from build123d import *

# Parameters (mm, degrees)
F1_DEPTH = 38.1
F3_DEPTH = 60.292894
F5_R     = 5.25769
F5_W     = 14.030187
F5_H     = 4.162106
F6_DEPTH = 130.254248
F4_W     = 54.139016
F4_H     = 9.669455
F7_DEPTH = 60.292894


with BuildPart() as f1:
    # F0 (on Top) → F1 (new body)
    with BuildSketch(Plane.XY):
        Polygon((82.095571, 21.614075), (-48.157677, 21.614075), (-48.157677, -38.677819), (36.971442, -38.677819), (36.971442, -20.666091), (82.095571, -20.666091), align=None)
    extrude(amount=F1_DEPTH)

    # F2 (on face) → F3 (cut, through all)
    with BuildSketch(Plane.XZ.offset(38.677819)):
        Polygon((82.158446, 38.1), (28.353805, 38.1), (82.158446, 0), align=None)
    extrude(amount=-F3_DEPTH, mode=Mode.SUBTRACT)

    # F5 (on face) → F6 (cut, through all)
    with BuildSketch(Plane(origin=(-48.157677, 0, 0), x_dir=(0, -1, 0), z_dir=(-1, 0, 0))):
        with Locations((-14.877267, 31.217162)):
            Circle(F5_R)
        with Locations((-2.21119, 31.217162)):
            Circle(F5_R)
        with Locations((-2.990069, 19.638609)):
            Circle(F5_R)
        with Locations((-14.2001, 19.638609)):
            Circle(F5_R)
        with Locations((12.323814, 36.018947)):
            Rectangle(F5_W, F5_H)
    extrude(amount=-F6_DEPTH, mode=Mode.SUBTRACT)

    # F4 (on face) → F7 (cut, through all)
    with BuildSketch(Plane.XZ.offset(38.677819)):
        with Locations((-21.088169, 4.834727)):
            Rectangle(F4_W, F4_H)
    extrude(amount=-F7_DEPTH, mode=Mode.SUBTRACT)


solid = f1.part
Could you check a few things on this model? Use its own coordinates, in mm. A direction names the side the tool comes from. Coordinates: 2 decimals unless noted, no trailing zeros. Order: outer loops, then holes, each group sorted by start corner. A loop starts at its lowest first (then second) coordinate and runs counter-clockwise, first axis right, second up. Notation, with made-up numbers: (37, 49.25) - (86, 49.25) arc R12 ccw to (86, 56.25) - close; hole circle Ø5 at (10.5, 76.5). An arc over 180 degrees is marked (long way). Answer in a Markdown table with one row per item. Add a question column.
(1) On a 3-axis mill with a long thin cutter (end or side, diameter ignored), from which of +Z, -Z, +X, -X, +Y, -Y can I reach the whole of each face in a straight line? I mean faces 1 (the face through (54, -20.666, 12)), 2 (the face through (-21, -9, 9.669)), 3 (the face through (-8, -19.339, 36)). Say none if no direction works.
(2) Will these pins go through, and if not, where does the flat tip stop? pin 1 (1 mm diameter, centred on y = 4, z = 7, fed in from +X); pin 2 (11 mm diameter, centred on x = -19.5, y = -13.5, fed in from +Z); pin 3 (1 mm diameter, centred on x = 53, z = 20, fed in from -Y).
(3) If we section it at B-B, the plane x = 43.5: Please give me the cut outline in (y, z), then the cut area to 3 significant figures.
(4) If we section it at A-A, the plane y = 0.5: Please give me the cut outline in (x, z).
(5) If we mould it in two halves opening along Y, with no side actions, what happens to faces 4 (the face through (-6, -38.678, 23)), 5 (the face through (6.163, 0.564, 14.974)), 6 (the face through (36.971, -30, 16)), 7 (the face through (6.163, 15.34, 14.506))? For each: released by +Y, released by -Y, zero draft, split by the parting line, or undercut.
(6) If we section it at D-D, the plane z = 30: Please give me the cut outline in (x, y), then the cut area to 3 significant figures.
(7) I need wall thicknesses on L1, parallel to Y at x = 29, z = 20; L2, parallel to Y at x = -16, z = 23; L3, parallel to Y at x = 2.5, z = 36. Which ranges of each line are inside material? Lowest first, please.
(8) If we section it at C-C, the plane y = -29: Please give me the cut outline in (x, z).
Results are:
| question | item | result |
|---|---|---|
| 1 | face 1 | +Z, -Z, +X, -Y |
| 1 | face 2 | -Z, -X, +Y, -Y |
| 1 | face 3 | +Z, +X, -X |
| 2 | pin 1 | stops at x = 72.98 |
| 2 | pin 2 | stops at z = 33.94 |
| 2 | pin 3 | stops at y = -20.67 |
| 3 | outline | (-20.67, 0) - (21.61, 0) - (21.61, 27.37) - (18.47, 27.37) arc R5.26 cw to (11.29, 27.37) - (5.8, 27.37) arc R5.26 cw to (-1.38, 27.37) - (-20.67, 27.37) - close; hole circle Ø10.52 at (2.99, 19.64); hole circle Ø10.52 at (14.2, 19.64) |
| 3 | area | 970 mm2 |
| 4 | outline | (-48.16, 9.67) - (5.98, 9.67) - (5.98, 0) - (82.1, 0) - (82.1, 0.04) - (60.96, 15.01) - (-48.16, 15.01) - close; (-48.16, 24.27) - (47.89, 24.27) - (45.09, 26.25) - (-48.16, 26.25) - close; (-48.16, 36.19) - (31.05, 36.19) - (28.35, 38.1) - (-48.16, 38.1) - close |
| 5 | face 4 | released by -Y |
| 5 | face 5 | undercut |
| 5 | face 6 | zero draft |
| 5 | face 7 | undercut |
| 6 | outline | (-48.16, -38.68) - (36.97, -38.68) - (36.97, -20.67) - (39.79, -20.67) - (39.79, -2.9) - (-48.16, -2.9) - close; (-48.16, 7.33) - (39.79, 7.33) - (39.79, 9.76) - (-48.16, 9.76) - close; (-48.16, 19.99) - (39.79, 19.99) - (39.79, 21.61) - (-48.16, 21.61) - close |
| 6 | area | 3,450 mm2 |
| 7 | L1 | y = -38.68 to -2.26, 8.24 to 8.95, 19.45 to 21.61 |
| 7 | L2 | y = -38.68 to -1.05, 7.03 to 10.16, 18.24 to 21.61 |
| 7 | L3 | y = -38.68 to -19.34, -5.31 to 0.03, 4.39 to 12.69, 17.06 to 21.61 |
| 8 | outline | (-48.16, 9.67) - (5.98, 9.67) - (5.98, 0) - (36.97, 0) - (36.97, 32) - (28.35, 38.1) - (-48.16, 38.1) - close |
